Verification items for the finished model (mm, model axes). Face numbers are marked on the shaded views. Round coordinates to 2 decimals unless told otherwise and drop trailing zeros. Order: outer loops, then holes, each group sorted by start corner. A loop starts at its lowest first (then second) coordinate and runs counter-clockwise, first axis right, second up. Notation, with made-up numbers: M 62,71.25 L 108,71.25 A34 ccw 108,101.25 Z; hole C -31.5,-34 d1. An arc over 180 degrees is marked long. Answer as a JSON object with one key per item and string values. Group by question number.
Autodesk Inventor part; units mm, degrees
ref_plane "YZ Plane" through (0, 0, 0) normal (1, 0, 0) x (0, 1, 0)
ref_plane "XZ Plane" through (0, 0, 0) normal (0, 1, 0) x (-1, 0, 0)
ref_plane "XY Plane" through (0, 0, 0) normal (0, 0, 1) x (1, 0, 0)
sketch "Эскиз1" plane through (0, 0, 0) normal (0, 0, 1) x (1, 0, 0)
  line L0 (0, 5) -> (0, 0)
  line L1 (0, 0) -> (36, 0)
  line L2 (36, 0) -> (36, 20)
  line L3 (36, 20) -> (31, 20)
  line L4 (31, 20) -> (31, 5)
  line L5 (31, 5) -> (0, 5)
  dimension "d0" = 5
  dimension "d1" = 5
  dimension "d3" = 20
  dimension "d4" = 36
revolve "Вращение1" add sketch "Эскиз1" angle 360 about axis through (0, 5, 0) along (0, -1, 0)
sketch "Эскиз2" plane through (0, 0, 0) normal (1, 0, 0) x (0, 1, 0)
  line L0 (-4, 0) -> (24, 0)
  line L1 (0, -50.4) -> (0, 50.4)
  line L2 (0, 0) -> (0, 50)
  line L3 (0, 50) -> (10, 50)
  line L4 (10, 50) -> (10, 0)
  line L5 (0, 0) -> (10, 0)
  line L6 (20, 36) -> (0, 36)
  dimension "d6" = 10
  dimension "d7" = 50
revolve "Вращение2" add sketch "Эскиз2" angle 360 about axis through (0, -10, 0) along (0, 1, 0)
chamfer "Фаска1" distance 1 angle 45 1 edges at (0, 0, -50)
sketch "Эскиз3" plane through (0, 0, 0) normal (0, -1, 0) x (1, 0, 0)
  circle A0 centre (0, 0) radius 42.5 construction
  circle A1 centre (0, 42.5) radius 5.5
  line L0 (0, -70) -> (0, 70)
  line L1 (-70, 0) -> (70, 0)
  dimension "d10" = 85
  dimension "d9" = 11
hole "Отверстие1" at (0, 0, 42.5) direction (0, 1, 0) diameter 6.2 depth 15 tip angle 118 counterbore diameter 11 counterbore depth 6.8
pattern_circular "Круговой массив1" count 6 over 360 about axis through (0, -10, 0) along (0, 1, 0) of "Отверстие1"
sketch "Эскиз4" plane through (0, 20, 0) normal (0, 1, 0) x (1, 0, 0)
  circle A0 centre (0, 0) radius 36
  circle A1 centre (0, 0) radius 31
  circle A2 centre (0, 0) radius 31
  circle A3 centre (0, 0) radius 36
  dimension "d27" = 72
extrude "Выдавливание2" add sketch "Эскиз4" along normal blind 1
fillet "Сопряжение1" radius 1.3 1 edges at (-36, 10, 0)
sketch "Эскиз5" plane through (0, 21, 0) normal (0, 1, 0) x (1, 0, 0)
  circle A0 centre (0, 0) radius 31
  circle A1 centre (0, 0) radius 36
  point P0 (0, 0)
extrude "Выдавливание3" cut sketch "Эскиз5" against normal blind 3
chamfer "Фаска2" distance 2 angle 45 1 edges at (-36, 18, 0)
properties part number "Крышка большая_72"
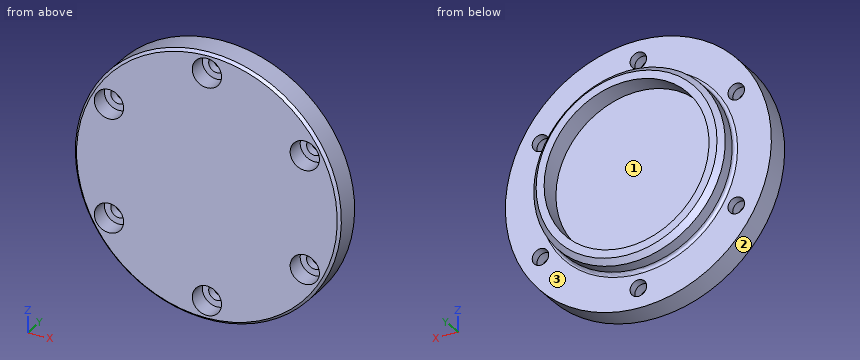
Q1. Release check for a two-part mould opening along Z. For the marked faces 1, 2 and 3 record: released by +Z, released by -Z, zero draft, split by the parting line, or undercut.
Q2. Cross-section at C-C, the plane y = 12.75. Record the cut outline in (x, z).
Q3. Thickness scan on line 1 (X direction, y = 9, z = -21.25); line 2 (Y direction, x = -7, z = 38.5); line 3 (X direction, y = 3.75, z = 39). Record the ranges inside material, lowest first. Write a range as from..to.
Q4. Gauge pin test, flat ends, axial feed: pin 1 Ø10 at (x, z) = (36.81, 21.25) entering from +Y; pin 2 Ø10 at (x, y) = (-23, 2) entering from -Z; pin 3 Ø10 at (x, z) = (-36.81, 21.25) entering from -Y. Record the tip position at first contact, or that the pin passes through.
Q5. Cross-section at B-B, the plane z = 0. Record the cut outline in (x, y).
Q6. Cross-section at D-D, the plane z = 21.25. Give the number of separate pieces and of enclosed holes in the cut face, then the cut area to 3 significant figures.
Q7. Cross-section at A-A, the plane y = 4. Record the cut outline in (x, z).
Conclusion:
{
 "1": {"face 1": "undercut", "face 2": "split by the parting line", "face 3": "zero draft"},
 "2": {"outline": "C 0,0 d72; hole C 0,0 d62"},
 "3": {"line 1": "-45.26..-39.91, -33.71..33.71, 39.91..45.26", "line 2": "0..10", "line 3": "-31.29..-4.24, 4.24..31.29"},
 "4": {"pin 1": "y = 10", "pin 2": "z = -46.65", "pin 3": "y = 6.8"},
 "5": {"outline": "M -50,1 L -49,0 L 49,0 L 50,1 L 50,10 L 37.3,10 A1.3 cw 36,11.3 L 36,16 L 34,18 L 31,18 L 31,10 L -31,10 L -31,18 L -34,18 L -36,16 L -36,11.3 A1.3 cw -37.3,10 L -50,10 Z"},
 "6": {"separate pieces": "3", "enclosed holes": "0", "area": "815 mm2"},
 "7": {"outline": "C 0,0 d100; hole C -36.81,-21.25 d11; hole C -36.81,21.25 d11; hole C 0,-42.5 d11; hole C 0,42.5 d11; hole C 36.81,-21.25 d11; hole C 36.81,21.25 d11"}
}
